Build history of the part. All positions in model axes, mm. Face numbers are marked on the shaded views. A direction names the side the tool comes from. Round coordinates to 2 decimals unless told otherwise and drop trailing zeros. Loops run counter-clockwise (first coordinate to the right, second up) from the corner with the lowest first, then second, coordinate; pieces in that order, holes last. Notation, with made-up numbers: (-7.5, 13.5) - (29.5, 13.5) arc R13 cw to (29.5, 33.5) - close; hole circle Ø7 at (57.25, -21.5). An arc over 180 degrees is marked (long way). Put each result on its own line as item: value. Start each with the question number.
from build123d import *

# Parameters (mm, degrees)
F0_W      = 90
F0_H      = 19.6
F0_W_2    = 15
F0_H_2    = 14
F0_W_3    = 20
F1_DEPTH  = 1
F2_W      = 17
F2_H      = 16
F2_W_2    = 15
F2_H_2    = 14
F2_W_3    = 22
F2_W_4    = 20
F3_DEPTH  = 13
F4_W      = 96
F4_H      = 25.6
F4_W_2    = 15
F4_H_2    = 14
F4_W_3    = 20
F5_DEPTH  = 1
F6_W      = 17
F6_H      = 2.5
F7_W      = 22
F7_H      = 2.5
F8_DEPTH  = 1.5
F10_W     = 17
F10_H     = 1.25
F10_W_2   = 22
F11_DEPTH = 10


with BuildPart() as f1:
    # F0 (on Top) → F1 (new body)
    with BuildSketch(Plane.XY):
        with Locations((45, 9.8)):
            Rectangle(F0_W, F0_H)
        with Locations((13.5, 11.6)):
            Rectangle(F0_W_2, F0_H_2, mode=Mode.SUBTRACT)
        with Locations((47, 11.6)):
            Rectangle(F0_W_3, F0_H_2, mode=Mode.SUBTRACT)
    extrude(amount=F1_DEPTH)

    # F2 (on face) → F3 (join)
    with BuildSketch(Plane(origin=(0, 0, 0), x_dir=(1, 0, 0), z_dir=(0, 0, -1))):
        with Locations((13.5, -11.6)):
            Rectangle(F2_W, F2_H)
        with Locations((13.5, -11.6)):
            Rectangle(F2_W_2, F2_H_2, mode=Mode.SUBTRACT)
        with Locations((47, -11.6)):
            Rectangle(F2_W_3, F2_H)
        with Locations((47, -11.6)):
            Rectangle(F2_W_4, F2_H_2, mode=Mode.SUBTRACT)
    extrude(amount=F3_DEPTH)

    # F4 (on Top) → F5 (join, through all)
    with BuildSketch(Plane.XY):
        with Locations((45, 9.8)):
            Rectangle(F4_W, F4_H)
        with Locations((13.5, 11.6)):
            Rectangle(F4_W_2, F4_H_2, mode=Mode.SUBTRACT)
        with Locations((47, 11.6)):
            Rectangle(F4_W_3, F4_H_2, mode=Mode.SUBTRACT)
    extrude(amount=F5_DEPTH)

    # F6 (on face) + F7 (on face) → F8 (join)
    with BuildSketch(Plane(origin=(0, 0, -13), x_dir=(1, 0, 0), z_dir=(0, 0, -1))):
        with Locations((13.5, -18.35)):
            Rectangle(F6_W, F6_H)
    with BuildSketch(Plane(origin=(0, 0, -13), x_dir=(1, 0, 0), z_dir=(0, 0, -1))):
        with Locations((47, -18.35)):
            Rectangle(F7_W, F7_H)
    extrude(amount=F8_DEPTH)

    # F10 (on 3pt) → F11 (join)
    with BuildSketch(Plane.XY.offset(-14.5)):
        with Locations((13.5, 17.725)):
            Rectangle(F10_W, F10_H)
        with Locations((47, 17.725)):
            Rectangle(F10_W_2, F10_H)
    extrude(amount=-F11_DEPTH)


solid = f1.part
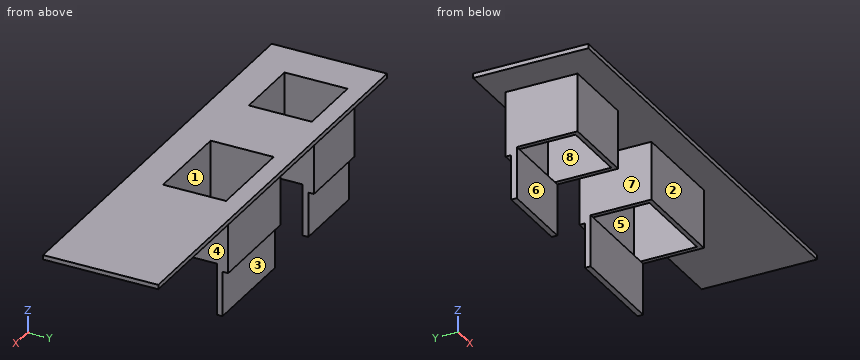
1) Slice it at D-D, the plane z = -18. Write the cut outline in (x, y).
2) Drill centre lines: line 1 (X direction, y = 17, z = -8.5); line 2 (X direction, y = 17.5, z = -19); line 3 (Y direction, x = 43, z = -5.5). Where is each one in solid material? Low to high. Write a range as [from, to].
3) Pull direction Y, two halves, no side cores. Call the marked faces 6, 7 and 8: pulls with the +Y half, pulls with the -Y half, needs draft (parallel to the pull), parting line crosses it, or undercut.
4) Slice it at C-C, the plane y = 14.25. Write the cut outline in (x, z), and give its area (3 significant figures).
5) Drop flat-ended pins along their axis: pin 1 Ø3 at (y, z) = (20, -14.5) entering from +X; pin 2 Ø12 at (x, z) = (45.5, -7) entering from +Y; pin 3 Ø1 at (x, z) = (12.5, -4.5) entering from -Y. Give the stop position or say it passes through.
6) Slice it at B-B, the plane x = 18.5. Write the cut outline in (y, z), and give its area (4 significant figures).
7) Which spindle directions (+Z, -Z, +X, -X, +Y, -Y) get a long thin tool onto all of the face, cutting with end or side? Do the marked faces 1, 2, 3, 4 and 5. Say none if no direction does.
8) Slice it at A-A, the plane z = -1.5. Write the cut outline in (x, y).
Taken from the geometry:
1. outline: (5, 17.1) - (22, 17.1) - (22, 18.35) - (5, 18.35) - close; (36, 17.1) - (58, 17.1) - (58, 18.35) - (36, 18.35) - close
2. line 1: x = [5, 6], [21, 22], [36, 37], [57, 58]
2. line 2: x = [5, 22], [36, 58]
2. line 3: y = [3.6, 4.6], [18.6, 19.6]
3. face 6: pulls with the -Y half
3. face 7: needs draft
3. face 8: undercut
4. outline: (-3, 0) - (5, 0) - (5, -13) - (6, -13) - (6, 1) - (-3, 1) - close; (21, -13) - (22, -13) - (22, 0) - (36, 0) - (36, -13) - (37, -13) - (37, 1) - (21, 1) - close; (57, -13) - (58, -13) - (58, 0) - (93, 0) - (93, 1) - (57, 1) - close
4. area: 113 mm2
5. pin 1: stops at x = 58
5. pin 2: stops at y = 19.6
5. pin 3: stops at y = 3.6
6. outline: (-3, 0) - (3.6, 0) - (3.6, -13) - (4.6, -13) - (4.6, 1) - (-3, 1) - close; (17.1, -24.5) - (18.35, -24.5) - (18.35, -14.5) - (19.6, -14.5) - (19.6, 0) - (22.6, 0) - (22.6, 1) - (18.6, 1) - (18.6, -13) - (17.1, -13) - close
6. area: 53.85 mm2
7. face 1: +Z, -Z
7. face 2: -Z, +X, -X, -Y
7. face 3: -Z, +X, -X, +Y
7. face 4: -Z, +X, +Y, -Y
7. face 5: +Z
8. outline: (5, 3.6) - (22, 3.6) - (22, 19.6) - (5, 19.6) - close; (36, 3.6) - (58, 3.6) - (58, 19.6) - (36, 19.6) - close; hole (6, 4.6) - (21, 4.6) - (21, 18.6) - (6, 18.6) - close; hole (37, 4.6) - (57, 4.6) - (57, 18.6) - (37, 18.6) - close
